```python
from build123d import *

# Parameters (mm, degrees)
SKETCH1_W            = 101.6
SKETCH1_H            = 53.3
BOSS_EXTRUDE1_DEPTH  = 3
SKETCH2_W            = 50
SKETCH2_H            = 4
SKETCH2_W_2          = 4
SKETCH2_H_2          = 48
SKETCH2_W_3          = 18
SKETCH2_H_3          = 10
SKETCH2_W_4          = 17.796210121
BOSS_EXTRUDE2_DEPTH  = 8
M3_CLEARANCE_HOLE1_D = 3.2


with BuildPart() as part:
    # Sketch1 → Boss-Extrude1 (new body)
    with BuildSketch(Plane(origin=(0, 0, 0), x_dir=(1, 0, 0), z_dir=(0, 1, 0))):
        with Locations((50.8, 26.65)):
            Rectangle(SKETCH1_W, SKETCH1_H)
    extrude(amount=BOSS_EXTRUDE1_DEPTH)

    # Sketch2 → Boss-Extrude2 (add)
    with BuildSketch(Plane(origin=(0, 3, 0), x_dir=(1, 0, 0), z_dir=(0, 1, 0))):
        with Locations((61.1, 49.8)):
            Rectangle(SKETCH2_W, SKETCH2_H)
        with Locations((98.1, 27.8)):
            Rectangle(SKETCH2_W_2, SKETCH2_H_2)
        with Locations((61.1, 3.5)):
            Rectangle(SKETCH2_W, SKETCH2_H)
        with Locations((4.5, 39.3)):
            Rectangle(SKETCH2_W_3, SKETCH2_H_3)
        with Locations((4.601894939, 14)):
            Rectangle(SKETCH2_W_4, SKETCH2_H_3)
    extrude(amount=BOSS_EXTRUDE2_DEPTH)

    # M3 Clearance Hole1 (through all)
    with Locations(Plane(origin=(0, 0, 0), x_dir=(-1, 0, 0), z_dir=(0, -1, 0))):
        with Locations((-14, 50.8), (-66.1, 45.7), (-66.1, 17.8), (-92.7, 50.8), (-15.3, 2.6), (-90.2, 2.6)):
            Hole(M3_CLEARANCE_HOLE1_D / 2)


solid = part.part
```
Input: part model. Units: mm. Frame: model coordinates. A direction names the side the tool comes from. Give positions to 0.01 mm unless a question says otherwise; leave off trailing zeros. Loops run counter-clockwise (first coordinate to the right, second up) from the corner with the lowest first, then second, coordinate; pieces in that order, holes last.
1) Mould query, pull axis X, two halves, no side actions, for faces 4 (the flat face through (61, 7, -5.5)), 5 (the flat face through (13.5, 7, -14)), 6 (the flat face through (-4.5, 7, -39)), 7 (the cylindrical face through (67.626, 1.521, -18.281)). Classes: released by +X, released by -X, zero draft, split by the parting line, or undercut.
A:
face 4: zero draft
face 5: undercut
face 6: released by -X
face 7: undercut
2) Section query C-C on x = 66.1. Return the cut outline in (y, z).
A:
outline: (0, -53.3) - (3, -53.3) - (3, -51.8) - (11, -51.8) - (11, -47.8) - (3, -47.8) - (3, -47.3) - (0, -47.3) - close; (0, -44.1) - (3, -44.1) - (3, -19.4) - (0, -19.4) - close; (0, -16.2) - (3, -16.2) - (3, -5.5) - (11, -5.5) - (11, -1.5) - (3, -1.5) - (3, 0) - (0, 0) - close
3) Reachability of faces 1 (the flat face through (13.5, 7, -39)), 2 (the flat face through (100.1, 7, -27)), 3 (the flat face through (36.1, 7, -3)) from +Z, -Z, +X, -X, +Y, -Y: full face, straight path, thin tool, end or side. Return the list, or none.
A:
face 1: +Z, -Z, +Y
face 2: +Z, -Z, +X, +Y
face 3: +Z, -Z, -X, +Y
4) Line query: L1, parallel to X at y = 1.3, z = -50.8; L2, parallel to Z at x = 66.1, y = 1.7; L3, parallel to X at y = 5.25, z = -11. Output: solid intervals per line, ascending.
A:
L1: x = 0 to 12.4, 15.6 to 91.1, 94.3 to 101.6
L2: z = -53.3 to -47.3, -44.1 to -19.4, -16.2 to 0
L3: x = -4.3 to 13.5, 96.1 to 100.1
5) Section query B-B on z = -50.8. Return the cut outline in (x, y).
A:
outline: (0, 0) - (12.4, 0) - (12.4, 3) - (0, 3) - close; (15.6, 0) - (91.1, 0) - (91.1, 3) - (86.1, 3) - (86.1, 11) - (36.1, 11) - (36.1, 3) - (15.6, 3) - close; (94.3, 0) - (101.6, 0) - (101.6, 3) - (100.1, 3) - (100.1, 11) - (96.1, 11) - (96.1, 3) - (94.3, 3) - close
6) Section query A-A on y = 7. Return the cut outline in (x, z), and give its area (3 significant figures).
A:
outline: (-4.5, -44.3) - (13.5, -44.3) - (13.5, -34.3) - (-4.5, -34.3) - close; (-4.3, -19) - (13.5, -19) - (13.5, -9) - (-4.3, -9) - close; (36.1, -51.8) - (86.1, -51.8) - (86.1, -47.8) - (36.1, -47.8) - close; (36.1, -5.5) - (86.1, -5.5) - (86.1, -1.5) - (36.1, -1.5) - close; (96.1, -51.8) - (100.1, -51.8) - (100.1, -3.8) - (96.1, -3.8) - close
area: 950 mm2
7) Section query D-D on z = -17.8. Return the cut outline in (x, y), and give its area (3 significant figures).
A:
outline: (-4.3, 3) - (0, 3) - (0, 0) - (64.5, 0) - (64.5, 3) - (13.5, 3) - (13.5, 11) - (-4.3, 11) - close; (67.7, 0) - (101.6, 0) - (101.6, 3) - (100.1, 3) - (100.1, 11) - (96.1, 11) - (96.1, 3) - (67.7, 3) - close
area: 470 mm2
8) Contact query for flat-ended pins moving along their axis: pin 1 (1.2 mm diameter, centred on x = 98.5, y = 5, fed in from +Z); pin 2 (2 mm diameter, centred on y = 7, z = -3, fed in from -X); pin 3 (2 mm diameter, centred on y = 7, z = -38.5, fed in from +X). Output: stop coordinate, or through.
A:
pin 1: stops at z = -3.8
pin 2: stops at x = 36.1
pin 3: stops at x = 100.1
